```python
from build123d import *

# Parameters (mm, degrees)
F0_W      = 50.3
F0_H      = 46.3
F0_R      = 1.5
F0_R_2    = 11.5
F1_DEPTH  = 4
F2_W      = 50.3
F2_H      = 4
F3_DEPTH  = 50
F5_DEPTH  = 3
F7_DEPTH  = 3
F9_DEPTH  = 4.001
F10_W     = 7
F10_H     = 47
F11_DEPTH = 2
F12_W     = 50.3
F12_H     = 23.15
F13_DEPTH = 54.001
F14_R     = 5


with BuildPart() as f1:
    # F0 (on Front) → F1 (new body)
    with BuildSketch(Plane.XZ):
        with Locations((0, 19.15)):
            Rectangle(F0_W, F0_H)
        with Locations((-15.5, 5.65)):
            Circle(F0_R, mode=Mode.SUBTRACT)
        with Locations((15.5, 5.65)):
            Circle(F0_R, mode=Mode.SUBTRACT)
        with Locations((-15.5, 36.65)):
            Circle(F0_R, mode=Mode.SUBTRACT)
        with Locations((0, 21.15)):
            Circle(F0_R_2, mode=Mode.SUBTRACT)
        with Locations((15.5, 36.65)):
            Circle(F0_R, mode=Mode.SUBTRACT)
    extrude(amount=F1_DEPTH)

    # F2 (on face) → F3 (join)
    with BuildSketch(Plane(origin=(0, 0, 0), x_dir=(-1, 0, 0), z_dir=(0, 1, 0))):
        with Locations((0, -2)):
            Rectangle(F2_W, F2_H)
    extrude(amount=F3_DEPTH)

    # F4 (on face) → F5 (join)
    with BuildSketch(Plane.YZ.offset(25.15)):
        Polygon((25, 0), (0, 21.15), (0, 0), align=None)
    extrude(amount=-F5_DEPTH)

    # F6 (on face) → F7 (join)
    with BuildSketch(Plane(origin=(-25.15, 0, 0), x_dir=(0, -1, 0), z_dir=(-1, 0, 0))):
        Polygon((0, 0), (0, 21.15), (-25, 0), align=None)
    extrude(amount=-F7_DEPTH)

    # F8 (on face) → F9 (cut, through all)
    with BuildSketch(Plane.XY):
        with BuildLine():
            Line((-14, 5), (-14, 45))
            ThreePointArc((-14, 45), (-15.5, 46.5), (-17, 45))
            Line((-17, 45), (-17, 5))
            ThreePointArc((-17, 5), (-15.5, 3.5), (-14, 5))
        make_face()
        with BuildLine():
            ThreePointArc((17, 45), (15.5, 46.5), (14, 45))
            Line((14, 45), (14, 5))
            ThreePointArc((14, 5), (15.5, 3.5), (17, 5))
            Line((17, 5), (17, 45))
        make_face()
    extrude(amount=-F9_DEPTH, mode=Mode.SUBTRACT)

    # F10 (on face) → F11 (cut)
    with BuildSketch(Plane.XY):
        with Locations((-15.5, 25)):
            Rectangle(F10_W, F10_H)
        with Locations((15.5, 25)):
            Rectangle(F10_W, F10_H)
    extrude(amount=-F11_DEPTH, mode=Mode.SUBTRACT)

    # F12 (on face) → F13 (cut, through all)
    with BuildSketch(Plane.XZ.offset(4)):
        with Locations((0, 30.725)):
            Rectangle(F12_W, F12_H)
    extrude(amount=-F13_DEPTH, mode=Mode.SUBTRACT)

    # F14
    f14_edges = [f1.edges().sort_by_distance(p)[0] for p in [
        (23.65, 2.364066, 19.15),
        (-23.65, 2.364066, 19.15),
        (11.324752, -2, 19.15),
        (-11.324752, -2, 19.15),
        (23.65, 25, 0),
        (-23.65, 25, 0),
        (25.15, 50, -2),
        (-25.15, 50, -2),
    ]]
    fillet(f14_edges, radius=F14_R)


solid = f1.part
```
Build history of the part. All positions in model axes, mm. A direction names the side the tool comes from. Coordinates: 2 decimals unless noted, no trailing zeros. Write each loop counter-clockwise with the first axis right and the second up, starting at its lowest first coordinate (ties: lowest second). Pieces come first, ordered by that corner, then holes.
1. Band-saw the part on B-B, the plane z = 5.65. Give the cut face in (x, y).
Answer block:
outline: (-25.15, -4) - (-17, -4) - (-17, 0) - (-22.15, 0) - (-22.15, 18.32) - (-25.15, 18.32) - close; (-14, -4) - (14, -4) - (14, 0) - (-14, 0) - close; (17, -4) - (25.15, -4) - (25.15, 18.32) - (22.15, 18.32) - (22.15, 0) - (17, 0) - close
2. Pull direction Z, two halves, no side cores. Call faces 1 (the flat face through (15, 48.5, -1)), 2 (the flat face through (0, 25, 0)), 3 (the cylindrical face through (14.39, -1.97, 6.66)): released by +Z, released by -Z, zero draft, split by the parting line, or undercut.
Answer block:
face 1: zero draft
face 2: released by +Z
face 3: undercut
3. Drill centre lines: probe 1 along X at (y, z) = (6, -2.25); probe 2 along Z at (x, y) = (15.5, -1.55); probe 3 along X at (y, z) = (5, 7.5). Where is each one in solid material? Low to high.
Answer block:
probe 1: x = -25.15 to -17, -14 to 14, 17 to 25.15
probe 2: z = -4 to 4.15, 7.15 to 19.15
probe 3: x = -25.15 to -22.15, 22.15 to 25.15
4. Band-saw the part on C-C, the plane z = 12. Give the cut face in (x, y), and give its area (3 significant figures).
Answer block:
outline: (-25.15, -4) - (-6.97, -4) - (-6.97, 0) - (-22.15, 0) - (-22.15, 10.82) - (-25.15, 10.82) - close; (6.97, -4) - (25.15, -4) - (25.15, 10.82) - (22.15, 10.82) - (22.15, 0) - (6.97, 0) - close
area: 210 mm2
5. Band-saw the part on D-D, the plane y = 6. Give the cut face in (x, z).
Answer block:
outline: (-25.15, -4) - (-17, -4) - (-17, -2) - (-19, -2) - (-19, 0) - (-22.15, 0) - (-22.15, 16.07) - (-25.15, 16.07) - close; (-14, -4) - (14, -4) - (14, -2) - (12, -2) - (12, 0) - (-12, 0) - (-12, -2) - (-14, -2) - close; (17, -4) - (25.15, -4) - (25.15, 16.07) - (22.15, 16.07) - (22.15, 0) - (19, 0) - (19, -2) - (17, -2) - close
6. Band-saw the part on A-A, the plane y = 15. Give the cut face in (x, z), and give its area (3 significant figures).
Answer block:
outline: (-25.15, -4) - (-17, -4) - (-17, -2) - (-19, -2) - (-19, 0) - (-22.15, 0) - (-22.15, 8.46) - (-25.15, 8.46) - close; (-14, -4) - (14, -4) - (14, -2) - (12, -2) - (12, 0) - (-12, 0) - (-12, -2) - (-14, -2) - close; (17, -4) - (25.15, -4) - (25.15, 8.46) - (22.15, 8.46) - (22.15, 0) - (19, 0) - (19, -2) - (17, -2) - close
area: 212 mm2
7. 3-axis set-ups, long thin cutter, end or side, ignore diameter. For faces 4 (the flat face through (-16, 48.5, -1)), 5 (the flat face through (-20, -2, 19.15)), 6 (the flat face through (14, 25, -3)), 7 (the cylindrical face through (-12.29, -1.97, 18.39)), 8 (the flat face through (22.15, 7, 8)): which of +Z, -Z, +X, -X, +Y, -Y reach the whole face in a straight line?
Answer block:
face 4: +Z
face 5: +Z, +X, -X, +Y, -Y
face 6: +Z, -Z
face 7: +Z, +Y, -Y
face 8: +Z, +Y
8. Drop flat-ended pins along their axis: pin 1 (1.5 mm diameter, centred on x = 15, y = 35.5, fed in from -Z); pin 2 (8 mm diameter, centred on x = -8, y = 1.5, fed in from +Z); pin 3 (4 mm diameter, centred on x = 15.5, z = 5.65, fed in from +Y). Give the stop position or say it passes through.
Answer block:
pin 1: passes through
pin 2: stops at z = 17.96
pin 3: stops at y = 0
